```python
from build123d import *

# Parameters (mm, degrees)
CYLINDER075_R     = 1.5
CYLINDER075_DEPTH = 50
CYLINDER076_R     = 1.5
CYLINDER076_DEPTH = 50
BOX001_W          = 20
BOX001_H          = 80
BOX001_DEPTH      = 60


with BuildPart() as cilindro075:
    # Cylinder075 → Cylinder075 (new body)
    with BuildSketch(Plane(origin=(-8, 8, 30), x_dir=(0, 0, -1), z_dir=(1, 0, 0))):
        Circle(CYLINDER075_R)
    extrude(amount=CYLINDER075_DEPTH)


with BuildPart() as fusion037:
    # Cylinder076 → Cylinder076 (new body)
    with BuildSketch(Plane(origin=(-8, 72, 30), x_dir=(0, 0, -1), z_dir=(1, 0, 0))):
        Circle(CYLINDER076_R)
    extrude(amount=CYLINDER076_DEPTH)

    # Fusion037: union Cilindro075
    add(cilindro075.part)


with BuildPart() as obj1:
    # Box001 → Box001 (new body)
    with BuildSketch(Plane.XY):
        with Locations((10, 40)):
            Rectangle(BOX001_W, BOX001_H)
    extrude(amount=BOX001_DEPTH)

    # Cut001: cut Fusion037
    add(fusion037.part, mode=Mode.SUBTRACT)


with BuildPart() as obj1_1:
    # Cut001 placement: moved
    add(obj1.part.moved(Location((19, -40, -11))))


solid = obj1_1.part
```
The model under review builds one solid part; all positions refer to its coordinate system, in mm. Round coordinates to 2 decimals unless told otherwise and drop trailing zeros. Loops run counter-clockwise (first coordinate to the right, second up) from the corner with the lowest first, then second, coordinate; pieces in that order, holes last. Notation, with made-up numbers: (-8, 72) - (14, 72) arc R27 ccw to (14, 92) - close; hole circle Ø4 at (55.25, -3.75). An arc over 180 degrees is marked (long way). Write each question's results on one line, items separated by ' | '. Start each with the question number.
Q1. Draft analysis for pull direction Y (two halves, no side actions). For faces 1 (the flat face through (29, 1, -11)), 2 (the flat face through (29, 40, 19)), 3 (the cylindrical face through (28.9, 31.1, 20.2)), state which applies: pulls with the +Y half, pulls with the -Y half, needs draft (parallel to the pull), parting line crosses it, or undercut.
Q2. Wall thickness on line 1 along Y through (x, z) = (26.25, 19); line 2 along Z through (x, y) = (33, 32): over which ranges is each line inside the solid? List them lowest first. Write a range as [from, to].
Q3. Take a section at B-B on z = 19. Give the boundary of the cut face in (x, y).
Q4. Take a section at A-A on y = 32. Give the boundary of the cut face in (x, z).
Q5. Insertion check: P1, Ø3.5, axis at y = -32, z = 19, coming from the +X side. The pin has a flat end and moves straight along its axis. Give the tip position at first contact, or say it passes through.
Data:
1) face 1: needs draft | face 2: pulls with the +Y half | face 3: undercut
2) line 1: y = [-40, -33.5], [-30.5, 30.5], [33.5, 40] | line 2: z = [-11, 17.5], [20.5, 49]
3) outline: (19, -40) - (39, -40) - (39, -33.5) - (19, -33.5) - close; (19, -30.5) - (39, -30.5) - (39, 30.5) - (19, 30.5) - close; (19, 33.5) - (39, 33.5) - (39, 40) - (19, 40) - close
4) outline: (19, -11) - (39, -11) - (39, 17.5) - (19, 17.5) - close; (19, 20.5) - (39, 20.5) - (39, 49) - (19, 49) - close
5) P1: stops at x = 39
